Part print with two shaded views. Sizes in mm from the minimum x, y, z corner. A direction names the side the tool comes from. Round coordinates to 2 decimals unless told otherwise and drop trailing zeros. Order: outer loops, then holes, each group sorted by start corner. A loop starts at its lowest first (then second) coordinate and runs counter-clockwise, first axis right, second up. Notation, with made-up numbers: (71.25, 32.5) -> (100.25, 32.5) arc R11 ccw to (100.25, 52.5) -> close; hole circle Ø4 at (-13.75, -10). An arc over 180 degrees is marked (long way). Use a Markdown table: item, result. Add a question column.
Item 1: Probe L1, parallel to X at y = 5.25, z = 5.5; L2, parallel to X at y = 11, z = 12.75; L3, parallel to Z at x = 36.5, y = 12.25. List the from-to ranges inside material, lowest first.
Item 2: Slice it at B-B, the plane z = 16.5. Give the cut face in (x, y).
Item 3: Two-plate mould, pull along X, no slides. Class the marked faces 6, 7, 8 and 9: released by +X, released by -X, zero draft, split by the parting line, or undercut.
Item 4: 3-axis set-ups, long thin cutter, end or side, ignore diameter. For the marked faces 1, 2, 3, 4 and 5: which of +Z, -Z, +X, -X, +Y, -Y reach the whole face in a straight line?
Item 5: Slice it at C-C, the plane x = 6.5. Give the cut face in (y, z) (3 decimals), plus the area to 3 significant figures.
Item 6: Slice it at D-D, the plane x = 33. Give the cut face in (y, z).
Item 7: Pin check, flat tips, straight feed: pin 1 (8 mm diameter, centred on x = 18.5, y = 9.5, fed in from +Z); pin 2 (0.5 mm diameter, centred on x = 5.5, z = 1, fed in from -Y) (3 decimals); pin 3 (0.8 mm diameter, centred on y = 5.5, z = 14, fed in from +X). Stop position of each tip, or through.
Item 8: Slice it at A-A, the plane y = 8. Give the cut face in (x, z).
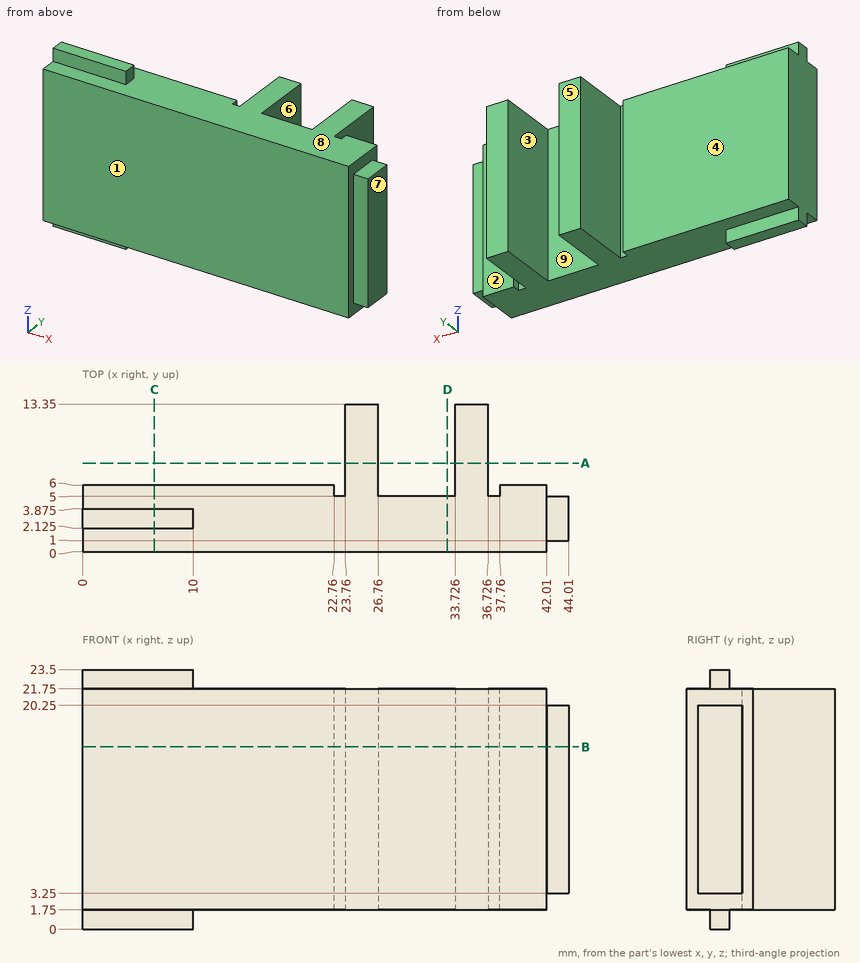
Check sheet entries:
| question | item | result |
|---|---|---|
| 1 | L1 | 0 to 22.76, 23.76 to 26.76, 33.73 to 36.73, 37.76 to 42.01 |
| 1 | L2 | 23.76 to 26.76, 33.73 to 36.73 |
| 1 | L3 | 1.75 to 21.75 |
| 2 | outline | (0, 0) -> (42.01, 0) -> (42.01, 1) -> (44.01, 1) -> (44.01, 5) -> (42.01, 5) -> (42.01, 6) -> (37.76, 6) -> (37.76, 5) -> (36.73, 5) -> (36.73, 13.35) -> (33.73, 13.35) -> (33.73, 5) -> (26.76, 5) -> (26.76, 13.35) -> (23.76, 13.35) -> (23.76, 5) -> (22.76, 5) -> (22.76, 6) -> (0, 6) -> close |
| 3 | face 6 | undercut |
| 3 | face 7 | released by +X |
| 3 | face 8 | zero draft |
| 3 | face 9 | undercut |
| 4 | face 1 | +Z, -Z, +X, -X, -Y |
| 4 | face 2 | +Z, -Z, +X, +Y |
| 4 | face 3 | +Z, -Z, +Y |
| 4 | face 4 | +Z, -Z, -X, +Y |
| 4 | face 5 | +Z, -Z, +X, -X, +Y |
| 5 | outline | (0, 1.75) -> (2.125, 1.75) -> (2.125, 0) -> (3.875, 0) -> (3.875, 1.75) -> (6, 1.75) -> (6, 21.75) -> (3.875, 21.75) -> (3.875, 23.5) -> (2.125, 23.5) -> (2.125, 21.75) -> (0, 21.75) -> close |
| 5 | area | 126 mm2 |
| 6 | outline | (0, 1.75) -> (5, 1.75) -> (5, 21.75) -> (0, 21.75) -> close |
| 7 | pin 1 | z = 21.75 |
| 7 | pin 2 | y = 2.125 |
| 7 | pin 3 | x = 42.01 |
| 8 | outline | (23.76, 1.75) -> (26.76, 1.75) -> (26.76, 21.75) -> (23.76, 21.75) -> close; (33.73, 1.75) -> (36.73, 1.75) -> (36.73, 21.75) -> (33.73, 21.75) -> close |
